Can you work these out from the model? Positions are in its coordinate system, mm. Face numbers are marked on the shaded views. A direction names the side the tool comes from. Give positions to 0.01 mm unless a question says otherwise; leave off trailing zeros. Write each loop counter-clockwise with the first axis right and the second up, starting at its lowest first coordinate (ties: lowest second). Pieces come first, ordered by that corner, then holes.
Solid Edge part; units mm, degrees
sketch "Sketch1" plane through (0, 0, 0) normal (0, 0, 1) x (1, 0, 0)
  line L0 (-23, -37.5) -> (23, -37.5)
  line L1 (23, -37.5) -> (23, 37.5)
  line L2 (23, 37.5) -> (-23, 37.5)
  line L3 (-23, 37.5) -> (-23, -37.5)
extrude "Protrusion1" add sketch "Sketch1" against normal blind 17
sketch "Sketch2" plane through (0, 0, 0) normal (0, 0, 1) x (1, 0, 0)
  arc A0 (-9.3209, -6.2097) -> (-9.3209, 6.2097) centre (0, 0) cw
  line L0 (-11.0309, 7.9196) -> (-9.3209, 6.2097)
  arc A1 (-11.0309, 7.9196) -> (-7.9196, 11.0309) centre (-9.4752, 9.4752) cw
  line L1 (-7.9196, 11.0309) -> (-6.2097, 9.3209)
  arc A2 (-6.2097, 9.3209) -> (6.2097, 9.3209) centre (0, 0) cw
  line L2 (7.9196, 11.0309) -> (6.2097, 9.3209)
  arc A3 (7.9196, 11.0309) -> (11.0309, 7.9196) centre (9.4752, 9.4752) cw
  line L3 (11.0309, 7.9196) -> (9.3209, 6.2097)
  arc A4 (9.3209, 6.2097) -> (9.3209, -6.2097) centre (0, 0) cw
  line L4 (11.0309, -7.9196) -> (9.3209, -6.2097)
  arc A5 (11.0309, -7.9196) -> (7.9196, -11.0309) centre (9.4752, -9.4752) cw
  line L5 (7.9196, -11.0309) -> (6.2097, -9.3209)
  arc A6 (6.2097, -9.3209) -> (-6.2097, -9.3209) centre (0, 0) cw
  line L6 (-7.9196, -11.0309) -> (-6.2097, -9.3209)
  arc A7 (-7.9196, -11.0309) -> (-11.0309, -7.9196) centre (-9.4752, -9.4752) cw
  line L7 (-11.0309, -7.9196) -> (-9.3209, -6.2097)
extrude "Cutout1" cut sketch "Sketch2" against normal through all
sketch "Sketch3" plane through (0, 37.5, -10) normal (0, 1, 0) x (-1, 0, 0)
  line L0 (-23, 10) -> (23, 10)
  line L1 (23, -7) -> (23, 10)
  line L2 (-23, -7) -> (23, -7)
  line L3 (-23, -7) -> (-23, 10)
extrude "ExtrudedProtrusion_2" add sketch "Sketch3" along normal blind 57
sketch "Sketch4" plane through (-23, 0, -10) normal (-1, 0, 0) x (0, -1, 0)
  circle A0 centre (28.5, 1.5) radius 4.2
  circle A1 centre (-85.5, 1.5) radius 4.2
extrude "Cutout2" cut sketch "Sketch4" against normal through all
sketch "Sketch5" plane through (-23, 0, -10) normal (-1, 0, 0) x (0, -1, 0)
  line L0 (-85.5, 1.5) -> (-88.5212, -1.4176)
  line L1 (-88.5212, -1.4176) -> (-85.5, -4.5461)
  line L2 (-85.5, -4.5461) -> (-82.4788, -1.4176)
  line L3 (-82.4788, -1.4176) -> (-85.5, 1.5)
  line L4 (28.5, 1.5) -> (25.4788, -1.4176)
  line L5 (25.4788, -1.4176) -> (28.5, -4.5461)
  line L6 (28.5, -4.5461) -> (31.5212, -1.4176)
  line L7 (31.5212, -1.4176) -> (28.5, 1.5)
extrude "Cutout3" cut sketch "Sketch5" against normal through all
sketch "Sketch6" plane through (0, 28.5, -17) normal (0, 0, -1) x (0, -1, 0)
  line L0 (-53.5, -23) -> (-53.5, 23)
  line L1 (-53.5, 23) -> (9.5, 23)
  line L2 (9.5, -23) -> (9.5, 23)
  line L3 (9.5, -23) -> (-53.5, -23)
extrude "ExtrudedProtrusion_4" add sketch "Sketch6" along normal blind 4.5
sketch "Sketch7" plane through (0, 28.5, -17) normal (0, 0, -1) x (0, -1, 0)
  line L0 (-66, 5) -> (-48, 5)
  line L1 (-48, 5) -> (18.8126, 23)
  dimension "D1" = 66
  dimension "D2" = 66
extrude "Cutout4" cut sketch "Sketch7" along normal through all and the other way through all material side at (-5.05, 85.5, -17)
sketch "Sketch8" plane through (0, 28.5, -17) normal (0, 0, -1) x (0, -1, 0)
  line L0 (-45.5, -7.3) -> (-19.5, -7.3)
  arc A0 (-19.5, -7.3) -> (-19.5, -11.7) centre (-19.5, -9.5) cw
  line L1 (-19.5, -11.7) -> (-45.5, -11.7)
  arc A1 (-45.5, -11.7) -> (-45.5, -7.3) centre (-45.5, -9.5) cw
  arc A2 (-8.5, 3.8) -> (-8.5, 8.2) centre (-8.5, 6) cw
  line L2 (-8.5, 8.2) -> (3.5, 8.2)
  arc A3 (3.5, 8.2) -> (3.5, 3.8) centre (3.5, 6) cw
  line L3 (3.5, 3.8) -> (-8.5, 3.8)
  circle A4 centre (0.5, -17) radius 2.2
extrude "Cutout5" cut sketch "Sketch8" along normal through all and the other way through all
sketch "Sketch9" plane through (0, -9.25, -17) normal (0, 0, -1) x (0, 1, 0)
  line L0 (-12.75, 18) -> (-12.75, -18)
  line L1 (25.25, -18) -> (-12.75, -18)
  line L2 (25.25, 18) -> (25.25, -18)
  line L3 (-12.75, 18) -> (25.25, 18)
  dimension "D1" = 12.75
  dimension "D2" = 25.25
  dimension "D3" = 12.75
extrude "ExtrudedCutout_8" cut sketch "Sketch9" against normal blind 10
fillet "Round_1" radius 5 4 edges at (18, 16, -12) (-18, 16, -12) (-18, -22, -12) (18, -22, -12)
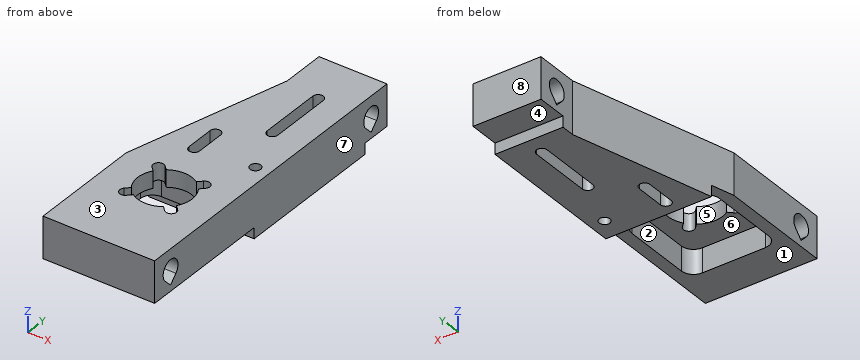
1) If we mould it in two halves opening along Y, with no side actions, what happens to the marked faces 6, 7 and 8? For each: +Y half, -Y half, draft (parallel to the pull), parting line (faces both ways), or undercut.
Values follow:
face 6: undercut
face 7: draft
face 8: +Y half
2) Please list where these lines run through material, in increasing order: L1, parallel to Y at x = 11.5, z = -7.5; L2, parallel to Y at x = 10.5, z = -8.5; L3, parallel to X at y = 28, z = -7.5.
Values follow:
L1: y = -37.5 to -32.58, -24.42 to -22, 16 to 47.08, 74.92 to 81.42, 89.58 to 94.5
L2: y = -37.5 to -32.7, -24.3 to -22, 16 to 46.04, 75.96 to 81.3, 89.7 to 94.5
L3: x = -18.07 to -8.2, -3.8 to 14.8, 19.2 to 23
3) Suppose I cut it at D-D on y = 28. Write out the boundary of the cut face in (x, z), plus the area to 3 significant figures.
Values follow:
outline: (-18.07, -21.5) - (-8.2, -21.5) - (-8.2, 0) - (-18.07, 0) - close; (-3.8, -21.5) - (14.8, -21.5) - (14.8, 0) - (-3.8, 0) - close; (19.2, -21.5) - (23, -21.5) - (23, 0) - (19.2, 0) - close
area: 694 mm2
4) Suppose I cut it at B-B on y = 52.5. Write out the boundary of the cut face in (x, z).
Values follow:
outline: (-11.47, -21.5) - (7.3, -21.5) - (7.3, 0) - (-11.47, 0) - close; (11.7, -21.5) - (23, -21.5) - (23, 0) - (11.7, 0) - close
5) Suppose I cut it at A-A on z = -8.5. State how many separate pieces and enclosed holes the cut face has, plus the area to 3 significant figures.
Values follow:
separate pieces: 3
enclosed holes: 4
area: 2,970 mm2
6) For the marked faces 1, 2, 3, 4 and 5, which set-ups out of +Z, -Z, +X, -X, +Y, -Y let a thin tool reach every point of the face, with its end or its side?
Values follow:
face 1: -Z, +X, -X, -Y
face 2: -Z
face 3: +Z, +X, -X, +Y, -Y
face 4: -Z, +X, -X, +Y
face 5: +Z, -Z
7) For pin 1 Ø5 at (y, z) = (50.5, -16.5) entering from -X; pin 2 Ø6 at (y, z) = (29.5, -7) entering from -X; pin 3 Ø11 at (y, z) = (64.5, -7) entering from -X, each with a flat end and sliding along its axis, tell me the tip position at first contact or that it passes through.
Values follow:
pin 1: stops at x = -12.68
pin 2: stops at x = -18.47
pin 3: stops at x = -9.71
